```python
from build123d import *

# Parameters (mm, degrees)
F0_R     = 50
F0_R_2   = 3.425
F0_W     = 7
F0_H     = 10
F0_R_3   = 30.5
F1_DEPTH = 10
F2_DEPTH = 25


# Not quite as in the source:
# - a feature names something its author has since deleted; it is built from what else it names


with BuildPart() as f1:
    # F0 (on Top) → F1 (new body)
    with BuildSketch(Plane.XY):
        Circle(F0_R)
        with Locations((-40.6804330647, -13.233267504)):
            Circle(F0_R_2, mode=Mode.SUBTRACT)
        with Locations((40.4436938465, -13.233267504)):
            Circle(F0_R_2, mode=Mode.SUBTRACT)
        with Locations((-40.547645092, 0.191732496)):
            Rectangle(F0_W, F0_H, mode=Mode.SUBTRACT)
        Circle(F0_R_3, mode=Mode.SUBTRACT)
        with Locations((40.3109058738, 0.191732496)):
            Rectangle(F0_W, F0_H, mode=Mode.SUBTRACT)
        with Locations((-40.6804330647, -13.233267504)):
            Circle(F0_R_2)
        with Locations((40.4436938465, -13.233267504)):
            Circle(F0_R_2)
    extrude(amount=F1_DEPTH)

    # F0 (on Top) → F2 (join)
    with BuildSketch(Plane.XY):
        with Locations((-40.6804330647, -13.233267504)):
            Circle(F0_R_2)
        with Locations((40.4436938465, -13.233267504)):
            Circle(F0_R_2)
    extrude(amount=F2_DEPTH)


solid = f1.part
```
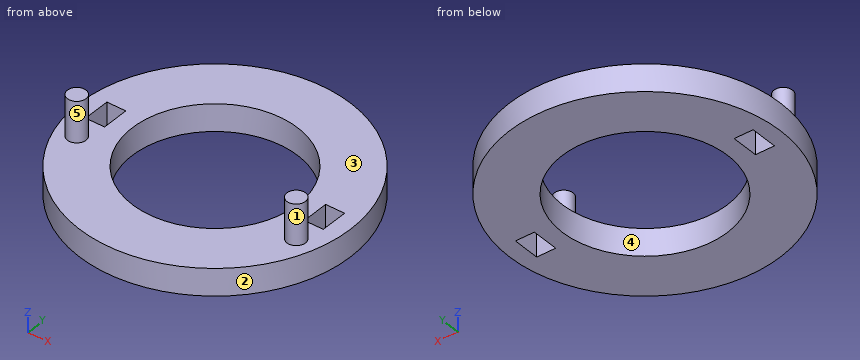
Geometry: final body of the model. Coordinates: model frame, mm. Face numbers are marked on the shaded views. A direction names the side the tool comes from. Coordinates: 2 decimals unless noted, no trailing zeros. Order: outer loops, then holes, each group sorted by start corner. A loop starts at its lowest first (then second) coordinate and runs counter-clockwise, first axis right, second up. Notation, with made-up numbers: M 46.5,86 L 67.5,86 A9 ccw 67.5,90 Z; hole C 79.25,-31.75 d11. An arc over 180 degrees is marked long. Answer in a Markdown table with one row per item. Add a question column.
Q1. Contact query for flat-ended pins moving along their axis: P1, Ø4, axis at x = 23.5, z = 6, coming from the +Y side; P2, Ø3.5, axis at x = -42, z = 5.5, coming from the -Y side; P3, Ø4, axis at y = -36.5, z = 8, coming from the -X side. Output: stop coordinate, or through.
Q2. Mould query, pull axis Y, two halves, no side actions, for the marked faces 3, 4 and 5. Classes: released by +Y, released by -Y, zero draft, split by the parting line, or undercut.
Q3. Line query: L1, parallel to X at y = -1, z = 5.5; L2, parallel to Y at x = 0, z = 7; L3, parallel to Z at x = -20, y = 40. Output: solid intervals per line, ascending.
Q4. Section query C-C on x = 0. Return the cut outline in (y, z).
Q5. Section query D-D on x = 17.5. Return the cut outline in (y, z).
Q6. Reachability of the marked faces 1 and 2 from +Z, -Z, +X, -X, +Y, -Y: full face, straight path, thin tool, end or side. Return the list, or none.
Q7. Section query A-A on z = 5. Return the cut outline in (x, y).
Q8. Section query B-B on y = 0. Return the cut outline in (x, z).
Completed:
| question | item | result |
|---|---|---|
| 1 | P1 | stops at y = 45.14 |
| 1 | P2 | stops at y = -29.66 |
| 1 | P3 | stops at x = -36.19 |
| 2 | face 3 | zero draft |
| 2 | face 4 | undercut |
| 2 | face 5 | split by the parting line |
| 3 | L1 | x = -49.99 to -44.05, -37.05 to -30.48, 30.48 to 36.81, 43.81 to 49.99 |
| 3 | L2 | y = -50 to -30.5, 30.5 to 50 |
| 3 | L3 | z = 0 to 10 |
| 4 | outline | M -50,0 L -30.5,0 L -30.5,10 L -50,10 Z; M 30.5,0 L 50,0 L 50,10 L 30.5,10 Z |
| 5 | outline | M -46.84,0 L -24.98,0 L -24.98,10 L -46.84,10 Z; M 24.98,0 L 46.84,0 L 46.84,10 L 24.98,10 Z |
| 6 | face 1 | +Z |
| 6 | face 2 | +Z, -Z |
| 7 | outline | C 0,0 d100; hole M -44.05,-4.81 L -37.05,-4.81 L -37.05,5.19 L -44.05,5.19 Z; hole C 0,0 d61; hole M 36.81,-4.81 L 43.81,-4.81 L 43.81,5.19 L 36.81,5.19 Z |
| 8 | outline | M -50,0 L -44.05,0 L -44.05,10 L -50,10 Z; M -37.05,0 L -30.5,0 L -30.5,10 L -37.05,10 Z; M 30.5,0 L 36.81,0 L 36.81,10 L 30.5,10 Z; M 43.81,0 L 50,0 L 50,10 L 43.81,10 Z |
